Geometry check sheet. Reference: drawing and pictorial views, mm from the part's lowest x, y, z. A direction names the side the tool comes from. Round coordinates to 2 decimals unless told otherwise and drop trailing zeros. Order: outer loops, then holes, each group sorted by start corner. A loop starts at its lowest first (then second) coordinate and runs counter-clockwise, first axis right, second up.
(1) Cross-section at B-B on x = 1.1. Enter the section's corners in (y, z) (1 decimal), and give its area (3 significant figures).
(2) Draft check along Z on the marked faces 1, 2 and 3. Enter one of: pulls with the +Z half, pulls with the -Z half, needs draft (parallel to the pull), parting line crosses it, or undercut.
(3) Set-up check for the marked faces 4 and 5: record each of +Z, -Z, +X, -X, +Y, -Y from which the full face is reachable in a straight line by a thin tool's end or side.
(4) Cross-section at C-C on x = 3.45. Enter the section's corners in (y, z).
(5) Cross-section at A-A on y = 3. Enter the section's corners in (x, z), and give its area (3 significant figures).
(6) Thickness scan on L1, parallel to X at y = 3, z = 3.55; L2, parallel to Z at x = 2.2, y = 2.95; L3, parallel to Y at x = 5.7, z = 2.1. Record the ranges inside material, lowest first.
(7) Gauge pin test, flat ends, axial feed: P1, Ø0.9, axis at x = 0.5, y = 3, coming from the -Z side; P2, Ø1, axis at x = 3.5, z = 2, coming from the -Y side; P3, Ø1.5, axis at x = 2, y = 1.5, coming from the +Z side; P4, Ø2, axis at x = 1, z = 2, coming from the -Y side. Record the tip position at first contact, or that the pin passes through.
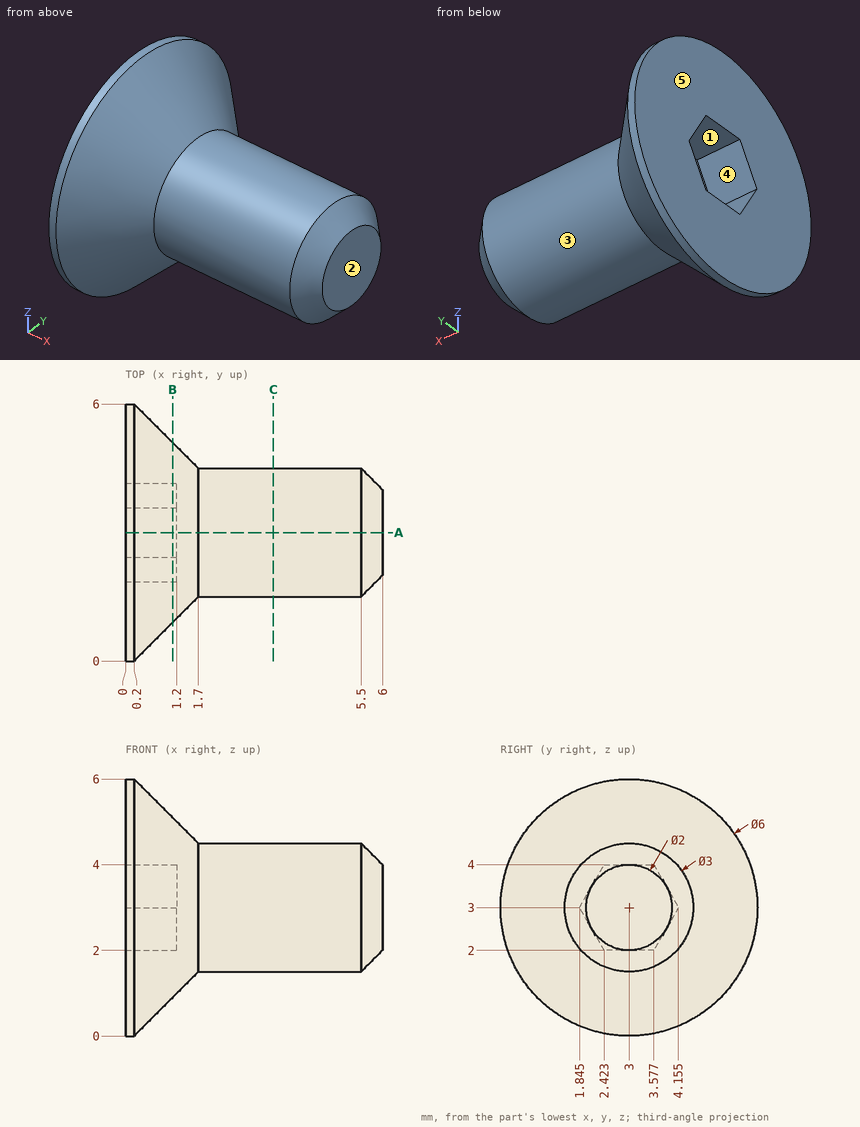
Found:
1. outline: circle Ø4.2 at (3, 3); hole (1.8, 3) - (2.4, 2) - (3.6, 2) - (4.2, 3) - (3.6, 4) - (2.4, 4) - close
1. area: 10.4 mm2
2. face 1: undercut
2. face 2: needs draft
2. face 3: parting line crosses it
3. face 4: -X
3. face 5: +Z, -Z, -X, +Y, -Y
4. outline: circle Ø3 at (3, 3)
5. outline: (0, 0) - (0.2, 0) - (1.7, 1.5) - (5.5, 1.5) - (6, 2) - (6, 4) - (5.5, 4.5) - (1.7, 4.5) - (0.2, 6) - (0, 6) - (0, 4) - (1.2, 4) - (1.2, 2) - (0, 2) - close
5. area: 18.2 mm2
6. L1: x = 1.2 to 6
6. L2: z = 1.5 to 4.5
6. L3: y = 2.06 to 3.94
7. P1: stops at z = 0
7. P2: stops at y = 1.59
7. P3: stops at z = 4.47
7. P4: stops at y = 0.03
